Build history of the part. All positions in model axes, mm. A direction names the side the tool comes from. Give positions to 0.01 mm unless a question says otherwise; leave off trailing zeros. Order: outer loops, then holes, each group sorted by start corner. A loop starts at its lowest first (then second) coordinate and runs counter-clockwise, first axis right, second up. Notation, with made-up numbers: (76, -15.5) -> (93, -15.5) arc R21 ccw to (93, 12.5) -> close; hole circle Ø3 at (77, -23). An arc over 180 degrees is marked (long way). One line per item, written item: value. Start each with the question number.
(1) Saw through at B-B on x = -38. Give the cut face in (y, z) (3 decimals), plus the area to 3 significant figures.
(2) Pin check, flat tips, straight feed: pin 1 (4 mm diameter, centred on x = 11.11, z = 58.74, fed in from -Y); pin 2 (1.3 mm diameter, centred on x = 53, y = 1.5, fed in from -Z) (3 decimals); pin 3 (1 mm diameter, centred on y = 1, z = 13.5, fed in from +X) (3 decimals). Stop position of each tip, or through.
(3) Saw through at A-A on z = 6.5. Give the cut face in (x, y) (3 decimals).
(4) Saw through at D-D on z = 18. Give the cut face in (x, y) (3 decimals), plus the area to 3 significant figures.
(5) Saw through at C-C on y = 0.4. Count the separate pieces of the cut face and the enclosed holes in it, plus the area to 3 significant figures.
(6) Two-plate mould, pull along Z, no slides. Class faces 3 (the flat face through (12, 0, 51)), 4 (the cylindrical face through (8.435, 1.252, 35.044)), 5 (the cylindrical face through (10.159, 1.252, 10.966)), 6 (the flat face through (-46, 1.3, 68.3)): +Z half, -Z half, draft (parallel to the pull), parting line (faces both ways), or undercut.
(7) Probe line 1 (X direction, y = 0.8, z = 56) (3 decimals); line 2 (X direction, y = 0.45, z = 60) (3 decimals); line 3 (Z direction, x = 52, y = 0.5) (3 decimals). List the from-to ranges inside material, lowest first.
(8) Which spindle directions (+Z, -Z, +X, -X, +Y, -Y) get a long thin tool onto all of the face, cutting with end or side? Do faces 1 (the flat face through (12, 2.54, 51)), 2 (the flat face through (22.225, 1, 13)). Say none if no direction does.
Autodesk Inventor part; units mm, degrees
ref_plane "YZ Plane" through (0, 0, 0) normal (1, 0, 0) x (0, 1, 0)
ref_plane "XZ Plane" through (0, 0, 0) normal (0, 1, 0) x (-1, 0, 0)
ref_plane "XY Plane" through (0, 0, 0) normal (0, 0, 1) x (1, 0, 0)
sketch "Sketch1" plane through (0, 0, 0) normal (0, 1, 0) x (-1, 0, 0)
  line L0 (-3.175, 0) -> (-19.05, 0)
  line L1 (-69.85, 50.8) -> (-69.85, 66.675)
  line L2 (-66.675, 69.85) -> (44.45, 69.85)
  line L3 (-66.675, 69.85) -> (-69.85, 66.675)
  line L4 (-22.225, 3.175) -> (-22.225, 22.225)
  line L5 (-47.625, 47.625) -> (-66.675, 47.625)
  arc A0 (-22.225, 22.225) -> (-47.625, 47.625) centre (-47.625, 22.225) ccw
  line L6 (-22.225, 3.175) -> (-19.05, 0)
  line L7 (-69.85, 50.8) -> (-66.675, 47.625)
  line L8 (0, 3.175) -> (0, 22.225)
  line L9 (25.4, 47.625) -> (44.45, 47.625)
  line L10 (47.625, 50.8) -> (47.625, 66.675)
  arc A1 (25.4, 47.625) -> (0, 22.225) centre (25.4, 22.225) ccw
  line L11 (44.45, 69.85) -> (47.625, 66.675)
  line L12 (44.45, 47.625) -> (47.625, 50.8)
  line L13 (-3.175, 0) -> (0, 3.175)
  point P0 (0, 0)
  point P1 (-69.85, 69.85)
  point P2 (-3.175, 0)
  point P3 (0, 0)
  point P4 (-22.225, 47.625)
  point P5 (-22.225, 0)
  point P6 (-69.85, 47.625)
  point P7 (52.01, 70.1655)
  point P8 (52.01, 44.7655)
  point P9 (5.867, 46.0375)
  point P10 (5.867, 11.0567)
  point P11 (0, 47.625)
  point P12 (41.275, 47.625)
  point P13 (47.625, 44.45)
  point P14 (47.625, 63.5)
  point P15 (47.625, 69.85)
  point P16 (47.625, 47.625)
  point P17 (0, 0)
  dimension "d6" = 3.175
  dimension "d7" = 3.175
  dimension "d10" = 25.4
  dimension "d11" = 3.175
  dimension "d12" = 3.175
  dimension "d13" = 3.175
  dimension "d14" = 3.175
  dimension "d39" = 19.05
  dimension "d40" = 19.05
  dimension "d44" = 22.225
  dimension "d45" = 25.4
  dimension "d46" = 3.175
  dimension "d47" = 3.175
  dimension "d48" = 3.175
  dimension "d49" = 3.175
  dimension "d50" = 19.05
  dimension "d56" = 22.225
  dimension "d57" = 22.225
  dimension "d58" = 3.175
  dimension "d59" = 3.175
extrude "Extrusion1" add sketch "Sketch1" along normal blind 2.54
hole "Hole1" at (11.1125, 2.54, 58.7375) direction (0, -1, 0) diameter 6.35 end through all
pattern_linear "Rectangular Pattern1" count 5 spacing 25.4 along (1, 0, 0) of "Hole1" first direction both ways yes
pattern_linear "Rectangular Pattern2" count 3 spacing 25.4 along (0, 0, -1) of "Hole1"
equation "\"d39\" = d50"
equation "\"d40\" = d50"
equation "\"d57\" = d44"
equation "\"BendRadius\" = Thickness"
equation "\"BendReliefWidth\" = Thickness"
equation "\"BendReliefDepth\" = 0.5 * Thickness"
equation "\"CornerReliefSize\" = 4 * Thickness"
equation "\"MinimumRemnant\" = 2 * Thickness"
equation "\"TransitionRadius\" = BendRadius"
equation "\"JacobiRadiusSize\" = Thickness"
equation "\"GapSize\" = Thickness"
properties part number "3x5 T"
Results below:
1. outline: (0, 47.625) -> (2.54, 47.625) -> (2.54, 56.048) -> (0, 56.048) -> close; (0, 61.427) -> (2.54, 61.427) -> (2.54, 69.85) -> (0, 69.85) -> close
1. area: 42.8 mm²
2. pin 1: passes through
2. pin 2: stops at z = 47.625
2. pin 3: stops at x = 22.225
3. outline: (0, 0) -> (8.282, 0) -> (8.282, 2.54) -> (0, 2.54) -> close; (13.943, 0) -> (22.225, 0) -> (22.225, 2.54) -> (13.943, 2.54) -> close
4. outline: (0, 0) -> (22.225, 0) -> (22.225, 2.54) -> (0, 2.54) -> close
4. area: 56.5 mm²
5. separate pieces: 1
5. enclosed holes: 7
5. area: 3,690 mm²
6. face 3: draft
6. face 4: undercut
6. face 5: undercut
6. face 6: +Z half
7. line 1: x = -47.625 to -41.296, -38.079 to -15.896, -12.679 to 9.504, 12.721 to 34.904, 38.121 to 60.304, 63.521 to 69.85
7. line 2: x = -47.625 to -42.601, -36.774 to -17.201, -11.374 to 8.199, 14.026 to 33.599, 39.426 to 58.999, 64.826 to 69.85
7. line 3: z = 47.625 to 69.85
8. face 1: +Z, -Z, +X, -X, +Y
8. face 2: -Z, +X, +Y, -Y
